Autodesk Inventor part; units mm, degrees
ref_plane "YZ Plane" through (0, 0, 0) normal (1, 0, 0) x (0, 1, 0)
ref_plane "XZ Plane" through (0, 0, 0) normal (0, 1, 0) x (-1, 0, 0)
ref_plane "XY Plane" through (0, 0, 0) normal (0, 0, 1) x (1, 0, 0)
sketch "Sketch1" plane through (0, 0, 0) normal (0, 0, 1) x (1, 0, 0)
  line L0 (2.1107, -2.6582) -> (2.6507, -2.6582)
  line L1 (2.6507, 2.3418) -> (2.1107, 2.3418)
  line L2 (-1.8893, -2.6582) -> (-1.8893, 2.3418)
  line L3 (-2.4293, -2.6582) -> (-1.8893, -2.6582)
  line L4 (-1.8893, 2.3418) -> (-2.4293, 2.3418)
  line L5 (2.6507, -4.6582) -> (2.6507, -2.6582)
  line L6 (2.6507, -4.6582) -> (1.9068, -4.6582)
  line L7 (0.1107, 4.3418) -> (-1.6853, 4.3418)
  line L8 (-2.4293, 2.3418) -> (-2.4293, 4.3418)
  line L9 (-1.6853, 4.3418) -> (-2.4293, 4.3418)
  line L10 (2.6507, -4.6582) -> (1.9068, -4.6582)
  line L11 (1.9068, -4.6582) -> (1.9068, 4.3418)
  line L12 (2.6507, 4.3418) -> (1.9068, 4.3418)
  line L13 (2.6507, 2.3418) -> (2.6507, 4.3418)
  line L14 (2.6507, 2.3418) -> (2.1107, 2.3418)
  line L15 (2.1107, 2.3418) -> (2.1107, -2.6582)
  line L16 (2.1107, -2.6582) -> (2.6507, -2.6582)
  line L17 (2.6507, -4.6582) -> (2.6507, -2.6582)
  line L18 (-1.6853, -4.6582) -> (-1.6853, 4.3418)
  line L19 (-1.6853, -4.6582) -> (-2.4293, -4.6582)
  line L20 (-2.4293, -4.6582) -> (-2.4293, -2.6582)
  line L21 (-2.4293, -2.6582) -> (-1.8893, -2.6582)
  line L22 (-1.8893, -2.6582) -> (-1.8893, 2.3418)
  line L23 (-1.8893, 2.3418) -> (-2.4293, 2.3418)
  line L24 (-2.4293, 2.3418) -> (-2.4293, 4.3418)
  line L25 (-1.6853, 4.3418) -> (-2.4293, 4.3418)
  line L26 (-1.6853, -4.6582) -> (-1.6853, 4.3418)
  line L27 (2.6507, -4.6582) -> (-2.4293, -4.6582)
  line L28 (2.1107, 2.3418) -> (2.1107, -2.6582)
  line L29 (-1.6853, -4.6582) -> (-2.4293, -4.6582)
  line L30 (2.6507, -4.6582) -> (-2.4293, -4.6582)
  line L31 (2.6507, -2.6582) -> (2.1107, -2.6582)
  line L32 (2.1107, -2.6582) -> (2.1107, 2.3418)
  line L33 (2.1107, 2.3418) -> (2.6507, 2.3418)
  line L34 (2.6507, 2.3418) -> (2.6507, 4.3418)
  line L35 (-2.4293, 4.3418) -> (2.6507, 4.3418)
  line L36 (-2.4293, 2.3418) -> (-2.4293, 4.3418)
  line L37 (-2.4293, 2.3418) -> (-1.8893, 2.3418)
  line L38 (-1.8893, 2.3418) -> (-1.8893, -2.6582)
  line L39 (-1.8893, -2.6582) -> (-2.4293, -2.6582)
  line L40 (-2.4293, -4.6582) -> (-2.4293, -2.6582)
  line L41 (2.6507, -4.6582) -> (-2.4293, -4.6582)
  line L42 (2.6507, -2.6582) -> (2.6507, -4.6582)
  line L43 (-1.3893, 4.3418) -> (1.6107, 4.3418)
  line L44 (1.9068, 4.3418) -> (0.1107, 4.3418)
  line L45 (0.1107, 4.3418) -> (-1.6853, 4.3418)
  line L46 (-1.6853, 4.3418) -> (-2.4293, 4.3418)
  line L47 (-2.4293, 4.3418) -> (2.6507, 4.3418)
  line L48 (2.6507, 4.3418) -> (1.9068, 4.3418)
  line L49 (2.6507, -4.6582) -> (-2.4293, -4.6582)
  line L50 (2.6507, -4.6582) -> (-2.4293, -4.6582)
  line L51 (2.6507, 2.3418) -> (2.6507, 4.3418)
  line L52 (2.1107, 2.3418) -> (2.6507, 2.3418)
  line L53 (2.6507, 2.3418) -> (2.6507, 4.3418)
  line L54 (2.6507, -2.6582) -> (2.1107, -2.6582)
  line L55 (2.6507, 2.3418) -> (2.6507, 4.3418)
  line L56 (2.6507, 2.3418) -> (2.6507, 4.3418)
  line L57 (2.6507, -2.6582) -> (2.6507, -4.6582)
  line L58 (2.6507, -4.6582) -> (2.6507, -2.6582)
  line L59 (2.6507, 2.3418) -> (2.1107, 2.3418)
  line L60 (2.1107, 2.3418) -> (2.6507, 2.3418)
  line L61 (2.1107, -2.6582) -> (2.6507, -2.6582)
  line L62 (2.6507, -2.6582) -> (2.1107, -2.6582)
  line L63 (2.1107, 2.3418) -> (2.1107, -2.6582)
  line L64 (2.1107, -2.6582) -> (2.1107, 2.3418)
  line L65 (-2.4293, -4.6582) -> (-2.4293, -2.6582)
  line L66 (2.6507, 4.3418) -> (1.9068, 4.3418)
  line L67 (-2.4293, 2.3418) -> (-2.4293, 4.3418)
  line L68 (-2.4293, -4.6582) -> (-2.4293, -2.6582)
  line L69 (-1.8893, -2.6582) -> (-2.4293, -2.6582)
  line L70 (-2.4293, 2.3418) -> (-1.8893, 2.3418)
  line L71 (-1.8893, -2.6582) -> (-1.8893, 2.3418)
  line L72 (-1.8893, 2.3418) -> (-1.8893, -2.6582)
  line L73 (-1.8893, -2.6582) -> (-2.4293, -2.6582)
  line L74 (-2.4293, -2.6582) -> (-1.8893, -2.6582)
  line L75 (-1.8893, 2.3418) -> (-2.4293, 2.3418)
  line L76 (-2.4293, 2.3418) -> (-1.8893, 2.3418)
  line L77 (-2.4293, -4.6582) -> (-2.4293, -2.6582)
  line L78 (-2.4293, -4.6582) -> (-2.4293, -2.6582)
  line L79 (-2.4293, 2.3418) -> (-2.4293, 4.3418)
  line L80 (-2.4293, 2.3418) -> (-2.4293, 4.3418)
  line L81 (-2.4293, 4.3418) -> (2.6507, 4.3418)
  line L82 (-1.8893, 2.3418) -> (-1.8893, -2.6582)
  line L83 (2.6507, -2.6582) -> (2.6507, -4.6582)
  line L84 (1.9068, -4.6582) -> (1.9068, 4.3418)
  line L85 (-1.3893, -3.6582) -> (1.6107, -3.6582)
  line L86 (-1.3893, -3.6582) -> (1.6107, -3.6582)
  line L87 (-1.3893, 4.3418) -> (1.6107, 4.3418)
  line L88 (-1.3893, -3.6582) -> (1.6107, -3.6582)
  line L89 (-1.3893, 4.3418) -> (1.6107, 4.3418)
  line L90 (2.1107, -2.6582) -> (2.1107, 2.3418)
  line L91 (1.9068, 4.3418) -> (0.1107, 4.3418)
  line L92 (2.6507, 2.8418) -> (-2.4293, 2.8418)
  line L93 (2.6507, 2.8418) -> (-2.4293, 2.8418)
  line L94 (-2.4293, 2.8418) -> (2.6507, 2.8418)
  line L95 (2.6507, 2.8418) -> (-2.4293, 2.8418)
  point P0 (0, 0)
  point P1 (0.1107, 2.8418)
  point P2 (0.1107, 2.8418)
  point P3 (0.1107, 2.8418)
  point P4 (-2.4293, 2.8418)
  point P5 (2.6507, 2.8418)
  point P6 (2.6507, 2.8418)
  point P7 (0.1107, 2.8418)
  point P8 (0.1107, 2.8418)
  point P9 (0.1107, 2.8418)
  point P10 (0.1107, 2.8418)
extrude "Extrusion1" add sketch "Sketch1" along normal blind 27
sketch "Sketch2" plane through (-2.4293, 4.3418, 0) normal (0, 1, 0) x (1, 0, 0)
  line L0 (0, -27) -> (5.08, -27)
  circle A0 centre (2.4293, -5.14) radius 1.5
  point P0 (2.4293, 0)
  point P1 (2.54, -27)
  point P2 (2.4293, 0)
  dimension "d2" = 21.86
  dimension "d3" = 3
extrude "Extrusion2" cut sketch "Sketch2" against normal blind 27
sketch "Sketch3" plane through (-2.4293, -4.6582, 0) normal (0, -1, 0) x (1, 0, 0)
  line L0 (5.08, 27) -> (0, 27)
  line L1 (2.54, 27) -> (2.4293, 0)
  circle A0 centre (2.5277, 24) radius 1
  circle A1 centre (2.5031, 18) radius 1
  dimension "d6" = 2
  dimension "d7" = 2
  dimension "d8" = 3
  dimension "d9" = 9
  dimension "d10" = 5.08
extrude "Extrusion3" cut sketch "Sketch3" against normal blind 27
properties part number "UpperGripperfingerpart_3DPrint"
Geometry: final body of the model. Coordinates: model frame, mm. A direction names the side the tool comes from. Round coordinates to 2 decimals unless told otherwise and drop trailing zeros. Loops run counter-clockwise (first coordinate to the right, second up) from the corner with the lowest first, then second, coordinate; pieces in that order, holes last.
Item 1: Mould query, pull axis Y, two halves, no side actions, for faces 1 (the flat face through (0, -4.658, 13)), 2 (the flat face through (0, 4.342, 13)), 3 (the flat face through (2.111, 0, 13)), 4 (the flat face through (2.651, -4, 13)). Classes: released by +Y, released by -Y, zero draft, split by the parting line, or undercut.
Checked values:
face 1: released by -Y
face 2: released by +Y
face 3: undercut
face 4: zero draft
Item 2: Line query: L1, parallel to Z at x = 0, y = 0.5; L2, parallel to Y at x = 2.45, z = 9.25; L3, parallel to Z at x = -0.6, y = -1. Output: solid intervals per line, ascending.
Checked values:
L1: z = 0 to 3.64, 6.64 to 17, 19 to 23, 25 to 27
L2: y = -4.66 to -2.66, 2.34 to 4.34
L3: z = 0 to 3.77, 6.51 to 17.26, 18.74 to 23.28, 24.72 to 27
Item 3: Section D-D, the plane z = 14.75. Output: boundary loops of the cut face in (x, y), plus the area to 3 significant figures.
Checked values:
outline: (-2.43, -4.66) - (2.65, -4.66) - (2.65, -2.66) - (2.11, -2.66) - (2.11, 2.34) - (2.65, 2.34) - (2.65, 4.34) - (-2.43, 4.34) - (-2.43, 2.34) - (-1.89, 2.34) - (-1.89, -2.66) - (-2.43, -2.66) - close
area: 40.3 mm2
Item 4: Reachability of faces 5 (the cylindrical face through (-0.143, -0.221, 17.024)), 6 (the flat face through (-1.889, 0, 13)) from +Z, -Z, +X, -X, +Y, -Y: full face, straight path, thin tool, end or side. Return the list, or none.
Checked values:
face 5: +Y, -Y
face 6: +Z, -Z, -X
Item 5: Section B-B, the plane x = 2.35. Output: boundary loops of the cut face in (y, z), plus the area to 3 significant figures.
Checked values:
outline: (-4.66, 0) - (-2.66, 0) - (-2.66, 27) - (-4.66, 27) - close; (2.34, 0) - (4.34, 0) - (4.34, 27) - (2.34, 27) - close
area: 108 mm2
Item 6: Section A-A, the plane z = 5.14. Output: boundary loops of the cut face in (x, y), plus the area to 3 significant figures.
Checked values:
outline: (-2.43, -4.66) - (-1.5, -4.66) - (-1.5, 4.34) - (-2.43, 4.34) - (-2.43, 2.34) - (-1.89, 2.34) - (-1.89, -2.66) - (-2.43, -2.66) - close; (1.5, -4.66) - (2.65, -4.66) - (2.65, -2.66) - (2.11, -2.66) - (2.11, 2.34) - (2.65, 2.34) - (2.65, 4.34) - (1.5, 4.34) - close
area: 13.3 mm2
Item 7: Contact query for flat-ended pins moving along their axis: P1, Ø2.5, axis at y = 0, z = 14, coming from the -X side; P2, Ø2.5, axis at x = 0.07, z = 18, coming from the -Y side; P3, Ø2.5, axis at y = 0, z = 7, coming from the +X side. Output: stop coordinate, or through.
Checked values:
P1: stops at x = -1.89
P2: stops at y = -4.66
P3: stops at x = 2.11
Item 8: Section C-C, the plane y = 1.75. Output: boundary loops of the cut face in (x, z), plus the area to 3 significant figures.
Checked values:
outline: (-1.89, 0) - (2.11, 0) - (2.11, 27) - (-1.89, 27) - close; hole circle Ø3 at (0, 5.14); hole circle Ø2 at (0.07, 18); hole circle Ø2 at (0.1, 24)
area: 94.6 mm2
